For this review, take the finished solid that the model builds, in its own axes (mm). A direction names the side the tool comes from. Round coordinates to 2 decimals unless told otherwise and drop trailing zeros. Write each loop counter-clockwise with the first axis right and the second up, starting at its lowest first coordinate (ties: lowest second). Pieces come first, ordered by that corner, then holes. Notation, with made-up numbers: (-39, 84.5) -> (5, 84.5) arc R22 ccw to (5, 115.5) -> close; hole circle Ø11 at (-27, -37). An arc over 180 degrees is marked (long way). Answer in a Markdown table with one row per item.
from build123d import *

# Parameters (mm, degrees)
SKETCH1_W           = 200
SKETCH1_H           = 10
BOSS_EXTRUDE1_DEPTH = 10
FILLET1_R           = 5
SKETCH2_R           = 2.5
CUT_EXTRUDE1_DEPTH  = 10
SKETCH3_W           = 10
SKETCH3_H           = 5
CUT_EXTRUDE2_DEPTH  = 10


with BuildPart() as part:
    # Sketch1 → Boss-Extrude1 (new body)
    with BuildSketch(Plane.XY):
        Rectangle(SKETCH1_W, SKETCH1_H)
    extrude(amount=BOSS_EXTRUDE1_DEPTH)

    # Fillet1
    fillet1_edges = [part.edges().sort_by_distance(p)[0] for p in [
        (-100, -5, 5),
        (-100, 5, 5),
        (100, -5, 5),
        (100, 5, 5),
    ]]
    fillet(fillet1_edges, radius=FILLET1_R - 0.0001)  # a hair under: the kernel refuses the full size

    # Sketch2 → Cut-Extrude1 (cut)
    with BuildSketch(Plane.XY.offset(10)):
        with Locations((95, 0)):
            Circle(SKETCH2_R)
        with Locations((-95, 0)):
            Circle(SKETCH2_R)
    extrude(amount=-CUT_EXTRUDE1_DEPTH, mode=Mode.SUBTRACT)

    # Sketch3 → Cut-Extrude2 (cut)
    with BuildSketch(Plane(origin=(0, 5, 0), x_dir=(1, 0, 0), z_dir=(0, 1, 0))):
        with Locations((-95, -5)):
            Rectangle(SKETCH3_W, SKETCH3_H)
        with Locations((95, -5)):
            Rectangle(SKETCH3_W, SKETCH3_H)
    extrude(amount=-CUT_EXTRUDE2_DEPTH, mode=Mode.SUBTRACT)


solid = part.part
1) Mouldability with a two-part tool opening along X and no side actions: class faces 1 (the cylindrical face through (-97.5, 0.1, 8.8)), 2 (the flat face through (-1, -5, 5)), 3 (the cylindrical face through (-99, -3, 9)) as pulls with the +X half, pulls with the -X half, needs draft (parallel to the pull), parting line crosses it, or undercut.
Solved:
| item | result |
|---|---|
| face 1 | undercut |
| face 2 | needs draft |
| face 3 | pulls with the -X half |
2) For line 1 (X direction, y = 0.25, z = 0.5); line 2 (Y direction, x = -95, z = 0.85); line 3 (X direction, y = -3.75, z = 3.25), list the stretches that pass through material, from the lowest coordinate up. Write a range as [from, to].
Solved:
| item | result |
|---|---|
| line 1 | [-99.99, -97.49], [-92.51, 92.51], [97.49, 99.99] |
| line 2 | [-5, -2.5], [2.5, 5] |
| line 3 | [-90, 90] |
3) Clearance check with flat-ended pins moving along their axes: pin 1 Ø4 at (y, z) = (-2, 6) entering from -X; pin 2 Ø4 at (x, y) = (95, 0) entering from -Z; pin 3 Ø1.5 at (y, z) = (-1.5, 5) entering from -X; pin 4 Ø2.5 at (y, z) = (1, 6) entering from +X. State where each tip first meets the part, or that it passes through.
Solved:
| item | result |
|---|---|
| pin 1 | x = -99.95 |
| pin 2 | through |
| pin 3 | x = -90 |
| pin 4 | x = 90 |
4) For faces 4 (the cylindrical face through (98, -4, 9)), 5 (the flat face through (93, 2, 7.5)), 6 (the flat face through (-92, 0, 7.5)), list the 3-axis set-ups (+Z, -Z, +X, -X, +Y, -Y) from which the entire face can be reached by the end or side of a thin tool; tool diameter is ignored.
Solved:
| item | result |
|---|---|
| face 4 | +Z, -Z, +X, -Y |
| face 5 | +X, +Y, -Y |
| face 6 | -X, +Y, -Y |
5) Consider section A-A on z = 4.5. State the section outline as (x, y) points, then the cut area to 3 significant figures.
Solved:
| item | result |
|---|---|
| outline | (-90, -5) -> (90, -5) -> (90, 5) -> (-90, 5) -> close |
| area | 1,800 mm² |
